```python
from build123d import *

# Parameters (mm, degrees)
F0_W     = 25.4
F0_H     = 25.4
F1_DEPTH = 3.175
F3_W     = 5.08
F3_H     = 12.7
F7_DEPTH = 6.35
F8_R     = 2.032
F9_DEPTH = 1.27


with BuildPart() as f1:
    # F0 (on Top) → F1 (new body)
    with BuildSketch(Plane.XY):
        Rectangle(F0_W, F0_H)
    extrude(amount=F1_DEPTH)



with BuildPart() as f4:
    # F4: sweep along a path in F2
    with BuildLine(Plane.XZ) as f4_path:
        ThreePointArc((-10.16, 0), (0, -23.5582897328), (10.16, 0))
    # F3 (on face) → F4 (sweep)
    with BuildSketch(Plane(origin=(0, 0, 0), x_dir=(1, 0, 0), z_dir=(0, 0, -1))):
        with Locations((10.16, 0)):
            Rectangle(F3_W, F3_H)
    sweep(path=f4_path.line)


with BuildPart() as f1_1:
    add(f1.part)

    add(f4.part)  # F7 merges F4
    # F6 (on Front) → F7 (join, symmetric)
    with BuildSketch(Plane.XZ):
        with BuildLine():
            ThreePointArc((-10.0130578512, -2.535746045), (-8.9072265211, -1.1822790439), (-7.62, 0))
            Line((-7.62, 0), (-10.16, 0))
            Line((-10.16, 0), (-10.0130578512, -2.535746045))
        make_face()
    extrude(amount=F7_DEPTH, both=True)

    # F8
    f8_edges = [f1_1.edges().sort_by_distance(p)[0] for p in [
        (-12.7, 0, 3.175),
        (12.7, 0, 3.175),
        (0, -12.7, 3.175),
        (0, 12.7, 3.175),
    ]]
    fillet(f8_edges, radius=F8_R)

    # F9 (cut): a face of the model
    f9_faces = [f1_1.faces().sort_by_distance(p)[0] for p in [
        (0, 0, 3.175),
    ]]
    extrude(f9_faces, amount=-F9_DEPTH, mode=Mode.SUBTRACT)


solid = f1_1.part
```
The listing builds one solid part. Answer for the finished solid, in the listing's coordinates (mm). A direction names the side the tool comes from. Round coordinates to 2 decimals unless told otherwise and drop trailing zeros. Loops run counter-clockwise (first coordinate to the right, second up) from the corner with the lowest first, then second, coordinate; pieces in that order, holes last.
Q1. Section B-B, the plane z = -4 is taken. Determine the outline of the cut face in (x, y).
Q2. Section C-C, the plane y = 0 is taken. Determine the outline of the cut face in (x, z) (3 decimals), then the cut area to 3 significant figures.
Q3. Given pin 1 Ø0.6 at (y, z) = (-4, 2.5) entering from +X; pin 2 Ø1 at (y, z) = (-2.5, -5) entering from +X; pin 3 Ø5 at (x, z) = (11.5, -18) entering from -Y, each flat-ended and moving along its own axis, determine where each tip first touches the part or whether it passes through.
Q4. Find the intervals of material crossed by line 1 (Z direction, x = -1, y = 3.25) (3 decimals); line 2 (Z direction, x = 4, y = 2) (3 decimals); line 3 (X direction, y = -1.75, z = -16.75), in increasing order.
Q5. Section D-D, the plane y = 9.25 is taken. Determine the outline of the cut face in (x, z) (3 decimals), then the cut area to 3 significant figures.
Q6. For a pull along Z with two mould halves and no side action, classify faces 6 (the face through (12.121, 0.178, 2.564)), 7 (the face through (-0.494, -0.089, -25.494)), 8 (the face through (-0.2, 12.7, 0.6)), 9 (the face through (0, 0, 0)) as released by +Z, released by -Z, zero draft, split by the parting line, or undercut.
Q7. Which of the six approach directions +Z, -Z, +X, -X, +Y, -Y give full straight-line access (tool end or side, diameter ignored) to faces 1 (the face through (0, 6.35, -22)), 2 (the face through (12.7, -0.2, 0.6)), 3 (the face through (0, 0, 1.905)), 4 (the face through (-12.7, -0.2, 0.6)), 5 (the face through (0, -6.35, -22))?
Q8. Section A-A, the plane x = 0 is taken. Determine the outline of the cut face in (y, z) (3 decimals), then the cut area to 3 significant figures.
Completed:
1. outline: (-14.9, -6.35) - (-10.9, -6.35) - (-10.9, 6.35) - (-14.9, 6.35) - close; (10.9, -6.35) - (14.9, -6.35) - (14.9, 6.35) - (10.9, 6.35) - close
2. outline: (-12.7, 0) arc R15.913 ccw (long way) to (12.7, 0) - (12.7, 1.143) arc R2.032 ccw to (10.668, 3.175) - (10.668, 1.905) - (-10.668, 1.905) - (-10.668, 3.175) arc R2.032 ccw to (-12.7, 1.143) - close; hole (-7.62, 0) arc R12.247 ccw (long way) to (7.62, 0) - close
2. area: 291 mm2
3. pin 1: stops at x = 12.4
3. pin 2: stops at x = 15.38
3. pin 3: stops at y = -6.35
4. line 1: z = -25.47 to -21.795, 0 to 1.905
4. line 2: z = -24.99 to -21.164, 0 to 1.905
4. line 3: x = -14.21 to -9.94, 9.94 to 14.21
5. outline: (-12.7, 0) - (12.7, 0) - (12.7, 1.143) arc R2.032 ccw to (10.668, 3.175) - (10.668, 1.905) - (-10.668, 1.905) - (-10.668, 3.175) arc R2.032 ccw to (-12.7, 1.143) - close
5. area: 51.8 mm2
6. face 6: released by +Z
6. face 7: split by the parting line
6. face 8: zero draft
6. face 9: undercut
7. face 1: -Z, +X, -X, +Y
7. face 2: +Z, +X, +Y, -Y
7. face 3: +Z
7. face 4: +Z, -X, +Y, -Y
7. face 5: -Z, +X, -X, -Y
8. outline: (-12.7, 0) - (12.7, 0) - (12.7, 1.143) arc R2.032 ccw to (10.668, 3.175) - (10.668, 1.905) - (-10.668, 1.905) - (-10.668, 3.175) arc R2.032 ccw to (-12.7, 1.143) - close; (-6.35, -25.501) - (6.35, -25.501) - (6.35, -21.836) - (-6.35, -21.836) - close
8. area: 98.3 mm2
